from build123d import *

# Parameters (mm, degrees)
F0_W      = 100
F0_H      = 80
F1_DEPTH  = 45
F5_R      = 7.5
F6_DEPTH  = 30
F8_DEPTH  = 80.001
F9_R      = 70
F10_DEPTH = 20
F11_W     = 20
F11_H     = 15
F12_DEPTH = 10
F14_DEPTH = 25.001


with BuildPart() as f1:
    # F0 (on Top) → F1 (new body)
    with BuildSketch(Plane.XY):
        with Locations((50, 40)):
            Rectangle(F0_W, F0_H)
    extrude(amount=F1_DEPTH)

    # F5 (on face) → F6 (cut, through all)
    with BuildSketch(Plane.XY.offset(45)):
        with Locations((60, 65)):
            Circle(F5_R)
    extrude(amount=-F6_DEPTH, mode=Mode.SUBTRACT)

    # F7 (on face) → F8 (cut, through all)
    with BuildSketch(Plane.XZ):
        with BuildLine():
            ThreePointArc((79.1062268166, 45), (94.5218269018, 24.8070038388), (100, 0))
            Line((100, 0), (100, 45))
            Line((100, 45), (79.1062268166, 45))
        make_face()
    extrude(amount=-F8_DEPTH, mode=Mode.SUBTRACT)

    # F9 (on face) → F10 (cut, through all)
    with BuildSketch(Plane.XY.offset(45)):
        Circle(F9_R)
    extrude(amount=-F10_DEPTH, mode=Mode.SUBTRACT)

    # F11 (on face) → F12 (join, through all)
    with BuildSketch(Plane.XY.offset(25)):
        with Locations((10, 7.5)):
            Rectangle(F11_W, F11_H)
    extrude(amount=F12_DEPTH)

    # F13 (on face) → F14 (cut, through all)
    with BuildSketch(Plane.XY.offset(25)):
        with BuildLine():
            Line((35, 30), (63.2455532034, 30))
            ThreePointArc((63.2455532034, 30), (51.4535762322, 47.4608206094), (35, 60.6217782649))
            Line((35, 60.6217782649), (35, 30))
        make_face()
    extrude(amount=-F14_DEPTH, mode=Mode.SUBTRACT)


solid = f1.part
The listing builds one solid part. Answer for the finished solid, in the listing's coordinates (mm). A direction names the side the tool comes from. Coordinates: 2 decimals unless noted, no trailing zeros. Order: outer loops, then holes, each group sorted by start corner. A loop starts at its lowest first (then second) coordinate and runs counter-clockwise, first axis right, second up.
Q1. Given P1, Ø6, axis at x = 41, z = 38, coming from the -Y side; P2, Ø12, axis at y = 36.5, z = 15.5, coming from the +X side; P3, Ø11, axis at y = 8, z = 32, coming from the +X side, each flat-ended and moving along its own axis, determine where each tip first touches the part or whether it passes through.
Q2. Consider line 1 (Y direction, x = 61, z = 17.5); line 2 (Z direction, x = 7.5, y = 43); line 3 (Y direction, x = 46.5, z = 15). Determine where each line is inside the solid, lowest interval first.
Q3. A cutting plane is placed at C-C, the plane y = 33. Write down the section's boundary in (x, z).
Q4. A cutting plane is placed at D-D, the plane z = 10.5. Write down the section's boundary in (x, y), and give its area (3 significant figures).
Q5. A cutting plane is placed at A-A, the plane z = 28. Write down the section's boundary in (x, y).
Q6. A cutting plane is placed at B-B, the plane x = 60. Write down the section's boundary in (y, z).
Q7. Which of the six approach directions +Z, -Z, +X, -X, +Y, -Y give full straight-line access (tool end or side, diameter ignored) to faces 1 (the face through (49, 30, 13)), 2 (the face through (10, 15, 30)), 3 (the face through (60, 65, 15)), 4 (the face through (10, 8, 35)), 5 (the face through (20, 7, 30))?
Q8. For a pull along Y with two mould halves and no side action, classify faces 6 (the face through (27, 28, 25)), 7 (the face through (35, 46, 13)), 8 (the face through (0, 39, 17)), 9 (the face through (49, 0, 17)) as pulls with the +Y half, pulls with the -Y half, needs draft (parallel to the pull), parting line crosses it, or undercut.
Answers follow:
1. P1: stops at y = 54.44
1. P2: stops at x = 99.23
1. P3: stops at x = 93.7
2. line 1: y = 0 to 30, 34.34 to 57.57, 72.43 to 80
2. line 2: z = 0 to 25
2. line 3: y = 0 to 30, 52.32 to 80
3. outline: (0, 0) - (35, 0) - (35, 25) - (0, 25) - close; (61.73, 0) - (100, 0) arc R58.91 ccw to (79.11, 45) - (61.73, 45) - close
4. outline: (0, 0) - (99.06, 0) - (99.06, 80) - (0, 80) - close; hole (35, 30) - (63.25, 30) arc R70 ccw to (35, 60.62) - close
4. area: 7,400 mm2
5. outline: (0, 0) - (20, 0) - (20, 15) - (0, 15) - close; (0, 70) arc R70 cw to (70, 0) - (92.92, 0) - (92.92, 80) - (0, 80) - close; hole circle Ø15 at (60, 65)
6. outline: (0, 0) - (30, 0) - (30, 25) - (0, 25) - close; (36.06, 0) - (80, 0) - (80, 45) - (72.5, 45) - (72.5, 15) - (57.5, 15) - (57.5, 45) - (36.06, 45) - close
7. face 1: +Z, -Z
7. face 2: +Z, -X
7. face 3: +Z
7. face 4: +Z, -X, -Y
7. face 5: +Z, -Y
8. face 6: undercut
8. face 7: undercut
8. face 8: needs draft
8. face 9: pulls with the -Y half
